Build history of the part. All positions in model axes, mm. Face numbers are marked on the shaded views. A direction names the side the tool comes from. Round coordinates to 2 decimals unless told otherwise and drop trailing zeros. Order: outer loops, then holes, each group sorted by start corner. A loop starts at its lowest first (then second) coordinate and runs counter-clockwise, first axis right, second up. Notation, with made-up numbers: (-32.75, -15.75) -> (-8.75, -15.75) arc R30 ccw to (-8.75, 18.25) -> close; hole circle Ø4 at (27, 74.25). An arc over 180 degrees is marked (long way). Write item = value, one per line.
from build123d import *

# Parameters (mm, degrees)
SKETCH_1_R          = 8
SKETCH_1_R_2        = 7.6
EXTRUDE_1_DEPTH     = 15
SKETCH_4_W          = 16
SKETCH_4_H          = 16
EXTRUDE_3_DEPTH     = 10
EXTRUDE_3_TAPER     = -45
SKETCH_6_W          = 36
SKETCH_6_H          = 36
EXTRUDE_5_DEPTH     = 15
SKETCH_7_W          = 32
SKETCH_7_H          = 32
CUT_EXTRUDE_3_DEPTH = 15
SKETCH_8_W          = 32
SKETCH_8_H          = 32
CUT_EXTRUDE_6_DEPTH = 9.2
CUT_EXTRUDE_6_DRAFT = -45
SKETCH_9_R          = 7.6
CUT_EXTRUDE_7_DEPTH = 40
SKETCH_10_W         = 3.2
SKETCH_10_H         = 36
EXTRUDE_7_DEPTH     = 3.2
SKETCH_11_R         = 0.6
CUT_EXTRUDE_8_DEPTH = 36


with BuildPart() as part:
    # Эскиз1 → Бобышка-Вытянуть1 (new body)
    with BuildSketch(Plane(origin=(0, 0, 0), x_dir=(0, 0, -1), z_dir=(1, 0, 0))):
        Circle(SKETCH_1_R)
        Circle(SKETCH_1_R_2, mode=Mode.SUBTRACT)
    extrude(amount=EXTRUDE_1_DEPTH)

    # Эскиз4 → Бобышка-Вытянуть3 (add)
    with BuildSketch(Plane(origin=(15, 0, 0), x_dir=(0, 0, -1), z_dir=(1, 0, 0))):
        Rectangle(SKETCH_4_W, SKETCH_4_H)
    extrude(amount=EXTRUDE_3_DEPTH, taper=EXTRUDE_3_TAPER)

    # Эскиз6 → Бобышка-Вытянуть5 (add)
    with BuildSketch(Plane(origin=(25, 0, 0), x_dir=(0, 0, -1), z_dir=(1, 0, 0))):
        Rectangle(SKETCH_6_W, SKETCH_6_H)
    extrude(amount=EXTRUDE_5_DEPTH)

    # Эскиз7 → Вырез-Вытянуть3 (cut)
    with BuildSketch(Plane(origin=(40, 0, 0), x_dir=(0, 0, -1), z_dir=(1, 0, 0))):
        Rectangle(SKETCH_7_W, SKETCH_7_H)
    extrude(amount=-CUT_EXTRUDE_3_DEPTH, mode=Mode.SUBTRACT)


with BuildPart() as cut_extrude_6_tool:
    # Эскиз8 → Вырез-Вытянуть6 (with draft: the straight prism first)
    with BuildSketch(Plane(origin=(25, 0, 0), x_dir=(0, 0, -1), z_dir=(1, 0, 0))):
        Rectangle(SKETCH_8_W, SKETCH_8_H)
    extrude(amount=-CUT_EXTRUDE_6_DEPTH)
    # Вырез-Вытянуть6: the draft: its side faces are tilted about the plane it starts from
    cut_extrude_6_sides = [cut_extrude_6_tool.faces().sort_by_distance(p)[0] for p in [
        (20.4, -16, 0),
        (20.4, 0, -16),
        (20.4, 16, 0),
        (20.4, 0, 16),
    ]]
    draft(cut_extrude_6_sides, Plane(origin=(25, 0, 0), x_dir=(0, 0, -1), z_dir=(1, 0, 0)), CUT_EXTRUDE_6_DRAFT)


with BuildPart() as part_1:
    add(part.part)

    # Вырез-Вытянуть6: cut by cut_extrude_6_tool
    add(cut_extrude_6_tool.part, mode=Mode.SUBTRACT)

    # Эскиз9 → Вырез-Вытянуть7 (cut)
    with BuildSketch(Plane.ZY):
        with Locations(Location((0, 0, 0), (0, 0, 26.525352017))):
            Circle(SKETCH_9_R)
    extrude(amount=-CUT_EXTRUDE_7_DEPTH, mode=Mode.SUBTRACT)

    # Эскиз10 → Бобышка-Вытянуть7 (add)
    with BuildSketch(Plane.XZ.offset(18)):
        with Locations((38.4, 0)):
            Rectangle(SKETCH_10_W, SKETCH_10_H)
    extrude(amount=EXTRUDE_7_DEPTH)

    # Эскиз11 → Вырез-Вытянуть8 (cut)
    with BuildSketch(Plane(origin=(0, 0, -18), x_dir=(-1, 0, 0), z_dir=(0, 0, -1))):
        with Locations((-38.4, -19.6)):
            Circle(SKETCH_11_R)
    extrude(amount=-CUT_EXTRUDE_8_DEPTH, mode=Mode.SUBTRACT)


solid = part_1.part
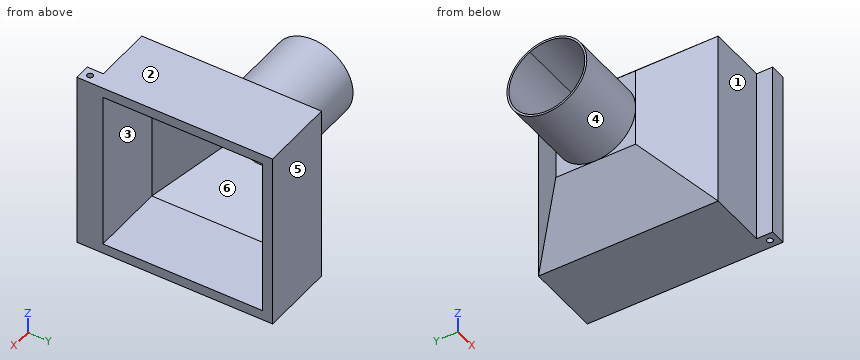
Q1. Flat gauge pins, fed straight in: pin 1 (3.5 mm diameter, centred on y = 5.5, z = 6, fed in from +X); pin 2 (1.5 mm diameter, centred on y = 6, z = 11.5, fed in from -X); pin 3 (6 mm diameter, centred on x = 17.5, z = 4, fed in from -Y); pin 4 (9 mm diameter, centred on y = 0, z = 0, fed in from -X). Where does each tip first touch, or does it go through?
Check values:
pin_1 = 16.75
pin_2 = 17.75
pin_3 = -13.5
pin_4 = through
Q2. Mould opens along Z. For the marked faces 4, 5 and 6 say: released by +Z, released by -Z, zero draft, split by the parting line, or undercut.
Check values:
face_4 = split by the parting line
face_5 = zero draft
face_6 = undercut
Q3. Cut at A-A, the plane x = 38.4. List the corners of the cut face in (y, z), and give its area (3 significant figures).
Check values:
outline = (-21.2, -18) -> (-20.2, -18) -> (-20.2, 18) -> (-21.2, 18) -> close; (-19, -18) -> (18, -18) -> (18, 18) -> (-19, 18) -> close; hole (-16, -16) -> (16, -16) -> (16, 16) -> (-16, 16) -> close
area = 344 mm²
Q4. Cut at B-B, the plane y = -19.6. List the corners of the cut face in (x, z), and give its area (3 significant figures).
Check values:
outline = (36.8, -18) -> (37.8, -18) -> (37.8, 18) -> (36.8, 18) -> close; (39, -18) -> (40, -18) -> (40, 18) -> (39, 18) -> close
area = 72.0 mm²
Q5. Which spindle directions (+Z, -Z, +X, -X, +Y, -Y) get a long thin tool onto all of the face, cutting with end or side? Do the marked faces 1, 2 and 3. Say none if no direction does.
Check values:
face_1 = +Z, -Z, -X, -Y
face_2 = +Z, +X, -X, +Y, -Y
face_3 = +X
Q6. Cut at D-D, the plane z = -5. Give the number of separate pieces and of enclosed holes in the cut face, and give its area (3 significant figures).
Check values:
separate_pieces = 2
enclosed_holes = 1
area = 126 mm²
Q7. Cut at C-C, the plane x = 26.5. List the corners of the cut face in (y, z).
Check values:
outline = (-18, -18) -> (18, -18) -> (18, 18) -> (-18, 18) -> close; hole (-16, -16) -> (16, -16) -> (16, 16) -> (-16, 16) -> close
Q8. Probe probe 1 along Y at (x, z) = (11, 0); probe 2 along Y at (x, z) = (38.4, -5); probe 3 along Y at (x, z) = (30.5, 14.5). List the from-to ranges inside material, lowest first.
Check values:
probe_1 = -8 to -7.6, 7.6 to 8
probe_2 = -21.2 to -20.2, -19 to -16, 16 to 18
probe_3 = -18 to -16, 16 to 18
